from build123d import *

# Parameters (mm, degrees)
ESQUISSE1_W             = 60
ESQUISSE1_H             = 15
ESQUISSE1_R             = 3.64432939
BOSS_EXTRU_2_DEPTH      = 10
BOSS_EXTRU_3_DEPTH      = 10
BOSS_EXTRU_3_DEPTH_BACK = 10
ESQUISSE2_R             = 1.5
ESQUISSE3_W             = 6.68566512
ESQUISSE3_H             = 5
ENL_V_MAT_EXTRU_1_DEPTH = 10
BOSS_EXTRU_5_DEPTH      = 10


with BuildPart() as part:
    # Esquisse1 → Boss.-Extru.2 (new body)
    with BuildSketch(Plane(origin=(0, 0, 0), x_dir=(1, 0, 0), z_dir=(0, 1, 0))):
        Rectangle(ESQUISSE1_W, ESQUISSE1_H)
        with Locations(Location((0, 0, 0), (0, 0, 270))):
            Circle(ESQUISSE1_R, mode=Mode.SUBTRACT)
    extrude(amount=BOSS_EXTRU_2_DEPTH)

    # Esquisse2 → Boss.-Extru.3 (add, two sides: drawn at the far end of the back side and taken through both)
    with BuildSketch(Plane(origin=(0, 0, 0), x_dir=(0, 0, -1), z_dir=(1, 0, 0)).offset(-BOSS_EXTRU_3_DEPTH_BACK)):
        with BuildLine():
            Line((-7.5, 0), (-32.699931919, 14.80760574))
            ThreePointArc((-32.699931919, 14.80760574), (-33.484005092, 15.654628224), (-33.66947754, 16.793846289))
            Line((-33.66947754, 16.793846289), (-33.012420508, 21.768308704))
            ThreePointArc((-33.012420508, 21.768308704), (-31.906962943, 23.303717227), (-30.016409528, 23.230754593))
            Line((-30.016409528, 23.230754593), (-7.5, 10))
            Line((-7.5, 10), (-7.5, 0))
        make_face()
        with Locations((-30.016409528, 18.484014396)):
            Circle(ESQUISSE2_R, mode=Mode.SUBTRACT)
    extrude(amount=BOSS_EXTRU_3_DEPTH + BOSS_EXTRU_3_DEPTH_BACK)

    # Esquisse3 → Enlèv. mat.-Extru.1 (cut)
    with BuildSketch(Plane(origin=(0, 10, 0), x_dir=(1, 0, 0), z_dir=(0, 1, 0))):
        Rectangle(ESQUISSE3_W, ESQUISSE3_H)
    extrude(amount=-ENL_V_MAT_EXTRU_1_DEPTH, mode=Mode.SUBTRACT)

    # Esquisse4 → Boss.-Extru.5 (add)
    with BuildSketch(Plane(origin=(0, 10, 0), x_dir=(1, 0, 0), z_dir=(0, 1, 0))):
        Polygon((-2.651629066, 2.5), (2.651629066, 2.5), (-0.901511212, 6.613696731), align=None)
        Polygon((-3.34283256, 1.451415578), (-3.34283256, -1.451415578), (-3.984232775, -1.229734519), (-3.663532667, 1.451415578), align=None)
        Polygon((3.34283256, 1.451415578), (3.34283256, -1.451415578), (4.44759228, -1.229734519), (3.971212027, 1.14433262), align=None)
        Polygon((2.651629066, -2.5), (-2.651629066, -2.5), (-2.371334481, -3.89686345), (1.661330759, -4.071090574), align=None)
    extrude(amount=-BOSS_EXTRU_5_DEPTH)


solid = part.part
Read the model definition and answer for the solid it produces. Units are mm, in the model's axes. A direction names the side the tool comes from. Coordinates: 2 decimals unless noted, no trailing zeros. Order: outer loops, then holes, each group sorted by start corner. A loop starts at its lowest first (then second) coordinate and runs counter-clockwise, first axis right, second up. Notation, with made-up numbers: (3, 6.5) - (42, 6.5) arc R14 cw to (42, 26.5) - close; hole circle Ø9 at (53.25, 5). An arc over 180 degrees is marked (long way). Use one line per item in the form item = value.
(1) Straight lines are drawn through the part: L1, parallel to X at y = 1.75, z = -0.5; L2, parallel to Y at x = 25, z = -6; L3, parallel to Z at x = -17, y = 8.75. For each, find the intervals that lie inside material, in ascending order.
Computed values:
L1 = -30 to -3.34, 3.34 to 30
L2 = 0 to 10
L3 = -7.5 to 7.5
(2) For a pull along X with two mould halves and no side action, classify faces 1 (the face through (10, 12, 20)), 2 (the face through (3.343, 5, 0)), 3 (the face through (-0.14, 7.3, 19.92)), 4 (the face through (0, 5, -2.5)) as pulls with the +X half, pulls with the -X half, needs draft (parallel to the pull), parting line crosses it, or undercut.
Computed values:
face_1 = pulls with the +X half
face_2 = undercut
face_3 = needs draft
face_4 = undercut
(3) Section C-C, the plane y = 1.5 is taken. Give the vertices of the cut face in (x, z), then the cut area to 3 significant figures.
Computed values:
outline = (-30, -7.5) - (30, -7.5) - (30, 7.5) - (10, 7.5) - (10, 10.05) - (-10, 10.05) - (-10, 7.5) - (-30, 7.5) - close; hole (-3.34, -2.5) - (3.34, -2.5) - (3.34, 2.5) - (-3.34, 2.5) - close
area = 918 mm²
(4) Which of the six approach directions +Z, -Z, +X, -X, +Y, -Y give full straight-line access (tool end or side, diameter ignored) to faces 5 (the face through (-0.14, 19.246, 33.346)), 6 (the face through (-20, 5, 7.5)), 7 (the face through (0, 5, 2.5)), 8 (the face through (0, 10, -3)), 9 (the face through (20, 5, 7.5))?
Computed values:
face_5 = +Z, +X, -X, +Y
face_6 = +Z, -X, +Y, -Y
face_7 = +Y, -Y
face_8 = -Z, +X, -X, +Y
face_9 = +Z, +X, +Y, -Y
(5) Section B-B, the plane y = 17.75 is taken. Give the vertices of the cut face in (x, z), then the cut area to 3 significant figures.
Computed values:
outline = (-10, 20.69) - (10, 20.69) - (10, 28.71) - (-10, 28.71) - close; (-10, 31.32) - (10, 31.32) - (10, 33.54) - (-10, 33.54) - close
area = 205 mm²
(6) Section A-A, the plane z = -1 is taken. Give the vertices of the cut face in (x, y), then the cut area to 3 significant figures.
Computed values:
outline = (-30, 0) - (-3.34, 0) - (-3.34, 10) - (-30, 10) - close; (3.34, 0) - (30, 0) - (30, 10) - (3.34, 10) - close
area = 533 mm²
(7) Section D-D, the plane x = 17.5 is taken. Give the vertices of the cut face in (y, z), then the cut area to 3 significant figures.
Computed values:
outline = (0, -7.5) - (10, -7.5) - (10, 7.5) - (0, 7.5) - close
area = 150 mm²
(8) Given pin 1 Ø7 at (y, z) = (15.5, 21.5) entering from -X; pin 2 Ø1.5 at (x, y) = (-14.5, 7.5) entering from +Z; pin 3 Ø5 at (y, z) = (18.48, 30.02) entering from +X, each flat-ended and moving along its own axis, determine where each tip first touches the part or whether it passes through.
Computed values:
pin_1 = -10
pin_2 = 7.5
pin_3 = 10
